Here's how the part is built. I have some questions about the finished solid (model axes, mm). Face numbers are marked on the shaded views. A direction names the side the tool comes from. Coordinates: 2 decimals unless noted, no trailing zeros. Write each loop counter-clockwise with the first axis right and the second up, starting at its lowest first coordinate (ties: lowest second). Pieces come first, ordered by that corner, then holes.
(1) Imagine slicing it at A-A, the plane y = 41. List the corners of the cut face in (x, z) for me.
(2) Thinking about a two-plate mould opening in Z: for the marked faces 6, 7, 8 and 9, which applies, released by +Z, released by -Z, zero draft, split by the parting line, or undercut?
(3) Please list where these lines run through material, in increasing order: probe 1 along Y at (x, z) = (4, -1); probe 2 along X at (y, z) = (10.5, -16); probe 3 along Z at (x, y) = (17.5, 4).
(4) Imagine slicing it at D-D, the plane z = -32. List the corners of the cut face in (x, y) for me, plus the area to 4 significant figures.
(5) Which directions (+Z, -Z, +X, -X, +Y, -Y) give clear straight access to the entire face, cutting with the end or side of a thin tool? Please do the marked faces 1, 2, 3, 4 and 5.
(6) For pin 1 Ø5 at (x, y) = (1, -4) entering from -Z; pin 2 Ø3.5 at (x, z) = (-14, 3.5) entering from +Y; pin 3 Ø16.5 at (x, z) = (10, 20) entering from +Y; pin 4 Ø12 at (x, z) = (9.5, -7.5) entering from +Y, each with a flat end and sliding along its axis, tell me the tip position at first contact or that it passes through.
(7) Imagine slicing it at B-B, the plane z = -16.5. List the corners of the cut face in (x, y) for me, plus the area to 3 significant figures.
(8) Imagine slicing it at C-C, the plane y = -0.75. List the corners of the cut face in (x, z) for me (3 decimals), plus the area to 3 significant figures.
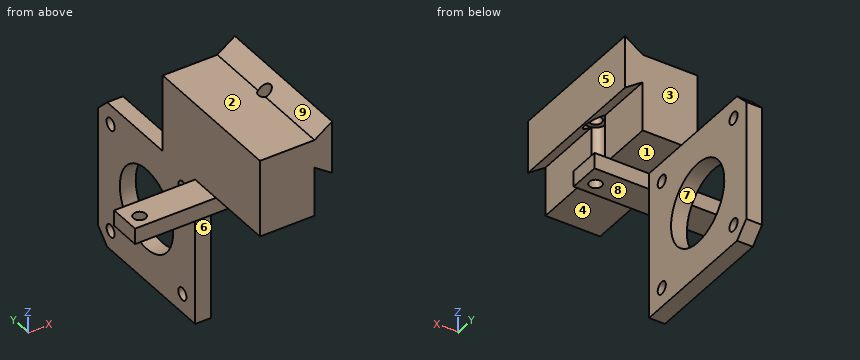
```python
from build123d import *

# Parameters (mm, degrees)
SKETCH_1_W            = 43
SKETCH_1_H            = 9
SKETCH_1_R            = 1.75
EXTRUDE_1_DEPTH       = 4.5
SKETCH_2_W            = 4.5
SKETCH_2_H            = 42
EXTRUDE_2_DEPTH       = 42
SKETCH_3_R            = 11.5
SKETCH_3_R_2          = 1.75
CUT_EXTRUDE_2_DEPTH   = 4.5
EXTRUDE_10_DEPTH      = 14
EXTRUDE_10_DEPTH_BACK = 28
SKETCH_11_W           = 5.5
SKETCH_11_H           = 22
SKETCH_1_6_R          = 1.75
CUT_EXTRUDE_7_DEPTH   = 64.659249132
CUT_EXTRUDE_START     = -4.5
SKETCH_12_R           = 3
CUT_EXTRUDE_8_DEPTH   = 14


with BuildPart() as part:
    # 草图1 → 凸台-拉伸1 (new body)
    with BuildSketch(Plane.XY):
        Rectangle(SKETCH_1_W, SKETCH_1_H)
        with Locations((-17.75, -0.75)):
            Circle(SKETCH_1_R, mode=Mode.SUBTRACT)
        with Locations(Location((17.75, -0.75, 0), (0, 0, 180))):
            Circle(SKETCH_1_R, mode=Mode.SUBTRACT)
    extrude(amount=EXTRUDE_1_DEPTH)

    # 草图2 → 凸台-拉伸2 (add)
    with BuildSketch(Plane.XY.offset(4.5)):
        with Locations((3.75, 25.5)):
            Rectangle(SKETCH_2_W, SKETCH_2_H)
    extrude(amount=-EXTRUDE_2_DEPTH)

    # 草图3 → 切除-拉伸2 (cut)
    with BuildSketch(Plane(origin=(6, 0, 0), x_dir=(0, 0, -1), z_dir=(1, 0, 0))):
        with Locations((16.5, 25.5)):
            Circle(SKETCH_3_R)
        with Locations((32, 41)):
            Circle(SKETCH_3_R_2)
        with Locations(Location((32, 10, 0), (0, 0, 180))):
            Circle(SKETCH_3_R_2)
        with Locations((1, 10)):
            Circle(SKETCH_3_R_2)
        with Locations(Location((1, 41, 0), (0, 0, 180))):
            Circle(SKETCH_3_R_2)
        Polygon((33.5, 46.5), (37.5, 42.5), (37.5, 46.5), align=None)
        Polygon((-0.5, 46.5), (-4.5, 42.5), (-4.5, 46.5), align=None)
    extrude(amount=-CUT_EXTRUDE_2_DEPTH, mode=Mode.SUBTRACT)

    # 草图11 → 凸台-拉伸10 (add, two sides: drawn at the far end of the back side and taken through both)
    with BuildSketch(Plane(origin=(0, 4.5, 0), x_dir=(1, 0, 0), z_dir=(0, 1, 0)).offset(-EXTRUDE_10_DEPTH_BACK)):
        Polygon((22, -22.5), (22, -15), (17, -18.5), (17, -22.5), align=None)
        Polygon((17, -22.5), (17, -18.5), (17, -4.5), (7, -4.5), (7, -26.5), (17, -26.5), align=None)
        Polygon((22, -30), (22, -22.5), (17, -22.5), (17, -26.5), align=None)
        with Locations((4.25, -15.5)):
            Rectangle(SKETCH_11_W, SKETCH_11_H)
    extrude(amount=EXTRUDE_10_DEPTH + EXTRUDE_10_DEPTH_BACK)

    # 草图1<6> → 切除-拉伸7 (cut, through all)
    with BuildSketch(Plane.XY):
        with Locations(Location((17.75, -0.75, 0), (0, 0, 180))):
            Circle(SKETCH_1_6_R)
    extrude(amount=CUT_EXTRUDE_7_DEPTH, mode=Mode.SUBTRACT)

    # 草图12 → 切除-拉伸8 (cut)
    with BuildSketch(Plane(origin=(0, 0, 0), x_dir=(-1, 0, 0), z_dir=(0, 0, -1)).offset(CUT_EXTRUDE_START)):
        with Locations((-17.75, -0.75)):
            Circle(SKETCH_12_R)
    extrude(amount=-CUT_EXTRUDE_8_DEPTH, mode=Mode.SUBTRACT)


solid = part.part
```
Recorded:
1. outline: (1.5, -37.5) - (6, -37.5) - (6, -33.75) - (1.5, -33.75) - close; (1.5, -30.25) - (6, -30.25) - (6, -2.75) - (1.5, -2.75) - close; (1.5, 0.75) - (6, 0.75) - (6, 4.5) - (1.5, 4.5) - close
2. face 6: zero draft
2. face 7: undercut
2. face 8: released by -Z
2. face 9: released by +Z
3. probe 1: y = 4.5 to 8.25, 11.75 to 39.25, 42.75 to 46.5
3. probe 2: x = 1.5 to 6
3. probe 3: z = 0 to 4.5, 18.15 to 26.85
4. outline: (1.5, 4.5) - (6, 4.5) - (6, 8.25) - (1.5, 8.25) - close; (1.5, 11.75) - (6, 11.75) - (6, 39.25) - (1.5, 39.25) - close; (1.5, 42.75) - (6, 42.75) - (6, 46.5) - (1.5, 46.5) - close
4. area: 157.5 mm2
5. face 1: -Z, +X, +Y
5. face 2: +Z, -X, +Y, -Y
5. face 3: +Z, +X, -X, +Y
5. face 4: -Z, +X, -X, -Y
5. face 5: +Z, -Z, +X, +Y, -Y
6. pin 1: stops at z = 0
6. pin 2: stops at y = 4.5
6. pin 3: stops at y = 18.5
6. pin 4: stops at y = 46.5
7. outline: (1.5, 4.5) - (6, 4.5) - (6, 14) - (1.5, 14) - close; (1.5, 37) - (6, 37) - (6, 46.5) - (1.5, 46.5) - close
7. area: 85.5 mm2
8. outline: (-21.5, 0) - (-19.5, 0) - (-19.5, 4.5) - (-21.5, 4.5) - close; (-16, 0) - (16, 0) - (16, 4.5) - (14.75, 4.5) - (14.75, 18.5) - (16, 18.5) - (16, 26.5) - (1.5, 26.5) - (1.5, 4.5) - (-16, 4.5) - close; (19.5, 0) - (21.5, 0) - (21.5, 4.5) - (19.5, 4.5) - close; (19.5, 18.5) - (20.75, 18.5) - (20.75, 15.875) - (22, 15) - (22, 30) - (19.5, 28.25) - close
8. area: 494 mm2
